Geometry: final body of the model. Coordinates: model frame, mm. Face numbers are marked on the shaded views. A direction names the side the tool comes from. Give positions to 0.01 mm unless a question says otherwise; leave off trailing zeros. Loops run counter-clockwise (first coordinate to the right, second up) from the corner with the lowest first, then second, coordinate; pieces in that order, holes last. Notation, with made-up numbers: (60.5, 18) - (85.5, 18) arc R28 ccw to (85.5, 41) - close; hole circle Ø8 at (55.25, 12.25). An arc over 180 degrees is marked (long way). Use CSV: the item, a comma, the result in double quotes. Start each with the question number.
```python
from build123d import *

# Parameters (mm, degrees)
SKETCH1_W           = 70.4
SKETCH1_H           = 44.6
BOSS_EXTRUDE1_DEPTH = 2
SKETCH3_R           = 1.65
CUT_EXTRUDE1_DEPTH  = 42.717262614
FILLET1_R           = 3
SKETCH4_W           = 30
SKETCH4_H           = 43
BOSS_EXTRUDE2_DEPTH = 30


with BuildPart() as part:
    # Sketch1 → Boss-Extrude1 (new body)
    with BuildSketch(Plane(origin=(0, 0, 0), x_dir=(1, 0, 0), z_dir=(0, 1, 0))):
        Rectangle(SKETCH1_W, SKETCH1_H)
    extrude(amount=BOSS_EXTRUDE1_DEPTH)

    # Sketch3 → Cut-Extrude1 (cut, through all)
    with BuildSketch(Plane(origin=(0, 2, 0), x_dir=(1, 0, 0), z_dir=(0, 1, 0))):
        with Locations(Location((-31.35, 18.8, 0), (0, 0, 270))):
            Circle(SKETCH3_R)
        with Locations(Location((31.35, 18.8, 0), (0, 0, 270))):
            Circle(SKETCH3_R)
        with Locations(Location((31.35, -18.8, 0), (0, 0, 270))):
            Circle(SKETCH3_R)
        with Locations(Location((-31.35, -18.8, 0), (0, 0, 270))):
            Circle(SKETCH3_R)
    extrude(amount=-CUT_EXTRUDE1_DEPTH, mode=Mode.SUBTRACT)

    # Fillet1
    fillet1_edges = [part.edges().sort_by_distance(p)[0] for p in [
        (35.2, 1, 22.3),
        (-35.2, 1, 22.3),
        (-35.2, 1, -22.3),
        (35.2, 1, -22.3),
    ]]
    fillet(fillet1_edges, radius=FILLET1_R)

    # Sketch4 → Boss-Extrude2 (add)
    with BuildSketch(Plane(origin=(0, 2, 0), x_dir=(1, 0, 0), z_dir=(0, 1, 0))):
        Rectangle(SKETCH4_W, SKETCH4_H)
    extrude(amount=BOSS_EXTRUDE2_DEPTH)


solid = part.part
```
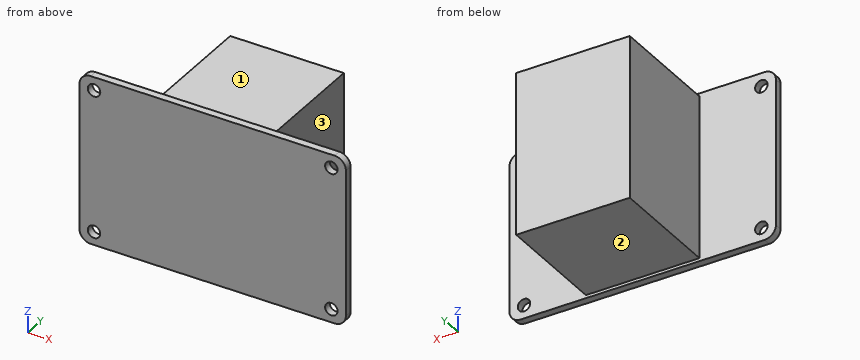
Item 1: Section C-C (x = -6.5). Output: boundary loops of the cut face in (y, z).
Item 2: Pin query (flat end, axial travel): pin 1 Ø3 at (x, y) = (13, 17.5) entering from +Z; pin 2 Ø2 at (x, z) = (31.35, 18.8) entering from -Y; pin 3 Ø9 at (x, y) = (-0.5, 19) entering from -Z; pin 4 Ø5 at (y, z) = (15, -4) entering from -X. Return the tip coordinate at first contact, or that it passes through.
Item 3: Ray query, probe 1 along X at (y, z) = (0.45, -18.8); probe 2 along Z at (x, y) = (31, 1); probe 3 along X at (y, z) = (1, -18). Return the intervals inside material, ascending.
Item 4: Section D-D (z = 8). Output: boundary loops of the cut face in (x, y), plus the area to 3 significant figures.
Item 5: Section A-A (x = -31.35). Output: boundary loops of the cut face in (y, z).
Item 6: Section B-B (z = -18). Output: boundary loops of the cut face in (x, y).
Item 7: Reachability of the marked faces 1, 2 and 3 from +Z, -Z, +X, -X, +Y, -Y: full face, straight path, thin tool, end or side. Return the list, or none.
Outcome:
1,outline,"(0, -22.3) - (2, -22.3) - (2, -21.5) - (32, -21.5) - (32, 21.5) - (2, 21.5) - (2, 22.3) - (0, 22.3) - close"
2,pin 1,"stops at z = 21.5"
2,pin 2,"passes through"
2,pin 3,"stops at z = -21.5"
2,pin 4,"stops at x = -15"
3,probe 1,"x = -35.2 to -33, -29.7 to 29.7, 33 to 35.2"
3,probe 2,"z = -22.3 to -20.41, -17.19 to 17.19, 20.41 to 22.3"
3,probe 3,"x = -35.2 to -32.79, -29.91 to 29.91, 32.79 to 35.2"
4,outline,"(-35.2, 0) - (35.2, 0) - (35.2, 2) - (15, 2) - (15, 32) - (-15, 32) - (-15, 2) - (-35.2, 2) - close"
4,area,"1,040 mm2"
5,outline,"(0, -22.3) - (2, -22.3) - (2, -20.45) - (0, -20.45) - close; (0, -17.15) - (2, -17.15) - (2, 17.15) - (0, 17.15) - close; (0, 20.45) - (2, 20.45) - (2, 22.3) - (0, 22.3) - close"
6,outline,"(-35.2, 0) - (-32.79, 0) - (-32.79, 2) - (-35.2, 2) - close; (-29.91, 0) - (29.91, 0) - (29.91, 2) - (15, 2) - (15, 32) - (-15, 32) - (-15, 2) - (-29.91, 2) - close; (32.79, 0) - (35.2, 0) - (35.2, 2) - (32.79, 2) - close"
7,face 1,"+Z, +X, -X, +Y"
7,face 2,"-Z, +X, -X, +Y"
7,face 3,"+Z, -Z, +X, +Y"
